Part model, mm, in its own coordinate system. Round coordinates to 2 decimals unless told otherwise and drop trailing zeros. Order: outer loops, then holes, each group sorted by start corner. A loop starts at its lowest first (then second) coordinate and runs counter-clockwise, first axis right, second up. Notation, with made-up numbers: (42, 65.5) -> (61, 65.5) arc R22 cw to (61, 101.5) -> close; hole circle Ø3 at (-31.5, 87). An arc over 180 degrees is marked (long way). Return JSON: item names as keys, results as strings. Group by question number.
from build123d import *

# Parameters (mm, degrees)
F0_W     = 279.4
F0_H     = 482.6
F0_W_2   = 19.951616
F0_H_2   = 26.186477
F0_W_3   = 19.951598
F0_W_4   = 155.703895
F0_H_3   = 30.60846
F0_W_5   = 19.220256
F0_H_4   = 37.062008
F1_DEPTH = 5


with BuildPart() as f1:
    # F0 (on Front) → F1 (new body)
    with BuildSketch(Plane.XZ):
        Rectangle(F0_W, F0_H)
        with Locations((-35.118891, 31.193768)):
            Rectangle(F0_W_2, F0_H_2, mode=Mode.SUBTRACT)
        with Locations((-0.203586, 31.193768)):
            Rectangle(F0_W_3, F0_H_2, mode=Mode.SUBTRACT)
        with Locations((0.261803, 115.733497)):
            Rectangle(F0_W_4, F0_H_3, mode=Mode.SUBTRACT)
        with Locations((112.11833, 18.531004)):
            Rectangle(F0_W_5, F0_H_4, mode=Mode.SUBTRACT)
        with Locations((0.261803, 164.973207)):
            Rectangle(F0_W_4, F0_H_3, mode=Mode.SUBTRACT)
    extrude(amount=F1_DEPTH)


solid = f1.part
(1) Probe L1, parallel to Z at x = -61.5, y = -1.65; L2, parallel to Z at x = -4, y = -4.2; L3, parallel to X at y = -2.4, z = 122.5. List the from-to ranges inside material, lowest first. Write a range as [from, to].
(2) Saw through at C-C, the plane x = -34.5. List the corners of the cut face in (y, z).
(3) Saw through at B-B, the plane y = -3.1. List the corners of the cut face in (x, z).
(4) Saw through at A-A, the plane x = 110. List the corners of the cut face in (y, z).
(5) Saw through at D-D, the plane x = -63. List the corners of the cut face in (y, z).
Results are:
{
 "1": {"L1": "z = [-241.3, 100.43], [131.04, 149.67], [180.28, 241.3]", "L2": "z = [-241.3, 18.1], [44.29, 100.43], [131.04, 149.67], [180.28, 241.3]", "L3": "x = [-139.7, -77.59], [78.11, 139.7]"},
 "2": {"outline": "(-5, -241.3) -> (0, -241.3) -> (0, 18.1) -> (-5, 18.1) -> close; (-5, 44.29) -> (0, 44.29) -> (0, 100.43) -> (-5, 100.43) -> close; (-5, 131.04) -> (0, 131.04) -> (0, 149.67) -> (-5, 149.67) -> close; (-5, 180.28) -> (0, 180.28) -> (0, 241.3) -> (-5, 241.3) -> close"},
 "3": {"outline": "(-139.7, -241.3) -> (139.7, -241.3) -> (139.7, 241.3) -> (-139.7, 241.3) -> close; hole (-77.59, 100.43) -> (78.11, 100.43) -> (78.11, 131.04) -> (-77.59, 131.04) -> close; hole (-77.59, 149.67) -> (78.11, 149.67) -> (78.11, 180.28) -> (-77.59, 180.28) -> close; hole (-45.09, 18.1) -> (-25.14, 18.1) -> (-25.14, 44.29) -> (-45.09, 44.29) -> close; hole (-10.18, 18.1) -> (9.77, 18.1) -> (9.77, 44.29) -> (-10.18, 44.29) -> close; hole (102.51, 0) -> (121.73, 0) -> (121.73, 37.06) -> (102.51, 37.06) -> close"},
 "4": {"outline": "(-5, -241.3) -> (0, -241.3) -> (0, 0) -> (-5, 0) -> close; (-5, 37.06) -> (0, 37.06) -> (0, 241.3) -> (-5, 241.3) -> close"},
 "5": {"outline": "(-5, -241.3) -> (0, -241.3) -> (0, 100.43) -> (-5, 100.43) -> close; (-5, 131.04) -> (0, 131.04) -> (0, 149.67) -> (-5, 149.67) -> close; (-5, 180.28) -> (0, 180.28) -> (0, 241.3) -> (-5, 241.3) -> close"}
}
